Answer from the drawing. Dimensions are ordinates in mm from the lowest x, y and z of the part. Coordinates: 2 decimals unless noted, no trailing zeros. Write each loop counter-clockwise with the first axis right and the second up, starting at its lowest first coordinate (ties: lowest second). Pieces come first, ordered by that corner, then holes. Notation, with made-up numbers: M 39.5,39.5 L 54.5,39.5 A16 ccw 54.5,46.5 Z; hole C 81.25,44 d6. An arc over 180 degrees is marked long. Put each result on its own line as item: value. Start each with the question number.
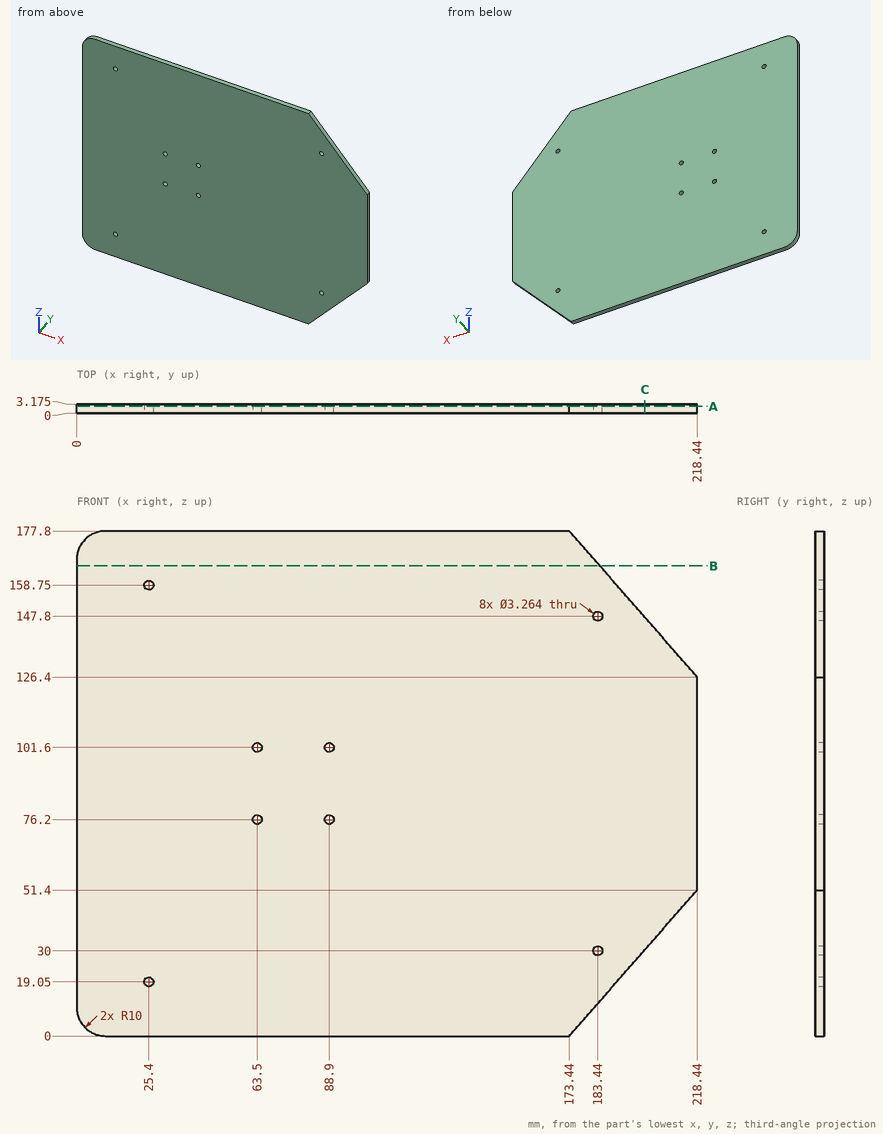
1) A cutting plane is placed at C-C on x = 200. Write down the section's boundary in (y, z) (1 decimal).
2) Given pin 1 Ø3 at (x, z) = (25.4, 158.75) entering from -Y, flat-ended and moving along its own axis, determine where the tip first touches the part or whether it passes through.
3) A cutting plane is placed at B-B on z = 165.5. Write down the section's boundary in (x, y) (1 decimal).
4) A cutting plane is placed at A-A on y = 2.3. State how many separate pieces and enclosed holes the cut face has, then the cut area to 3 significant figures.
5) Straight lines are drawn through the part: probe 1 along X at (y, z) = (0.7, 76.2); probe 2 along Z at (x, y) = (87.5, 0.9); probe 3 along X at (y, z) = (2, 147.8) (1 decimal). For each, find the intervals that lie inside material, in ascending order.
Answers follow:
1. outline: M 0,30.3 L 3.2,30.3 L 3.2,147.5 L 0,147.5 Z
2. pin 1: passes through
3. outline: M 0,0 L 184.2,0 L 184.2,3.2 L 0,3.2 Z
4. separate pieces: 1
4. enclosed holes: 8
4. area: 36,400 mm²
5. probe 1: x = 0 to 61.87, 65.13 to 87.27, 90.53 to 218.44
5. probe 2: z = 0 to 75.36, 77.04 to 100.76, 102.44 to 177.8
5. probe 3: x = 0 to 181.8, 185.1 to 199.7
